Geometry: final body of the model. Coordinates: model frame, mm. A direction names the side the tool comes from. Give positions to 0.01 mm unless a question says otherwise; leave off trailing zeros. Order: outer loops, then holes, each group sorted by start corner. A loop starts at its lowest first (then second) coordinate and runs counter-clockwise, first axis right, second up. Notation, with made-up numbers: (89, 84.25) - (105, 84.25) arc R20 ccw to (105, 115.25) - close; hole circle Ø4 at (-15, 74). An arc over 180 degrees is marked (long way). One line per item, written item: value.
Autodesk Inventor part; units mm, degrees
ref_plane "Work Plane1" through (-25.4, 0, -5.08) normal (0, 0, 1) x (1, 0, 0)
ref_plane "YZ Plane" through (0, 0, 0) normal (1, 0, 0) x (0, 1, 0)
ref_plane "XZ Plane" through (0, 0, 0) normal (0, 1, 0) x (-1, 0, 0)
sketch "Sketch1" plane through (0, 0, 0) normal (0, 1, 0) x (-1, 0, 0)
  point P0 (0, 0)
sketch "Sketch2" plane through (0, 0, 0) normal (0, 1, 0) x (-1, 0, 0)
  line L0 (0, 0) -> (25.4, 0)
  line L1 (25.4, 0) -> (25.4, -50.8)
  line L2 (25.4, -50.8) -> (0, -50.8)
  line L3 (0, -50.8) -> (0, 0)
  dimension "d0" = 25.4
  dimension "d1" = 50.8
extrude "Extrusion1" add sketch "Sketch2" along normal blind 25.4
sketch "Sketch3" plane through (-25.4, 0, 0) normal (0, 0, 1) x (1, 0, 0)
  line L0 (0, 25.4) -> (25.4, 25.4)
  line L1 (0, 0) -> (0, 25.4)
  line L2 (25.4, 0) -> (25.4, 25.4)
  line L3 (3.81, 21.59) -> (21.59, 21.59)
  line L4 (21.59, 21.59) -> (21.59, 15.24)
  line L5 (21.59, 15.24) -> (3.81, 15.24)
  line L6 (3.81, 15.24) -> (3.81, 21.59)
  line L7 (25.4, 0) -> (0, 0)
  line L8 (3.81, 3.81) -> (21.59, 3.81)
  line L9 (21.59, 3.81) -> (21.59, 10.16)
  line L10 (21.59, 10.16) -> (3.81, 10.16)
  line L11 (3.81, 10.16) -> (3.81, 3.81)
  dimension "d4" = 3.81
  dimension "d5" = 3.81
  dimension "d6" = 3.81
  dimension "d7" = 6.35
  dimension "d8" = 3.81
  dimension "d9" = 6.35
extrude "Extrusion2" cut sketch "Sketch3" against normal blind 5.08 contours L3 L4 L5 L6 | L11 L10 L9 L8
ref_plane "Work Plane1" through (-25.4, 0, -5.08) normal (0, 0, 1) x (1, 0, 0)
sketch "Sketch4" plane through (-25.4, 0, -5.08) normal (0, 0, 1) x (1, 0, 0)
  line L0 (2.54, 22.86) -> (22.86, 22.86)
  line L1 (22.86, 22.86) -> (22.86, 2.54)
  line L2 (22.86, 2.54) -> (2.54, 2.54)
  line L3 (2.54, 2.54) -> (2.54, 22.86)
  line L4 (0, 25.4) -> (25.4, 25.4)
  line L5 (0, 0) -> (0, 25.4)
  line L6 (25.4, 0) -> (25.4, 25.4)
  line L7 (25.4, 0) -> (0, 0)
  dimension "d13" = 2.54
  dimension "d14" = 2.54
  dimension "d15" = 2.54
  dimension "d16" = 2.54
extrude "Extrusion3" cut sketch "Sketch4" against normal blind 43.18 contours L0 L1 L2 L3
sketch "Sketch5" plane through (0, 0, -50.8) normal (0, 0, -1) x (-1, 0, 0)
  line L0 (2.54, 2.54) -> (22.86, 2.54)
  line L1 (9.525, 8.89) -> (15.875, 8.89)
  line L2 (15.875, 8.89) -> (15.875, 2.54)
  line L3 (15.875, 2.54) -> (9.525, 2.54)
  line L4 (9.525, 2.54) -> (9.525, 8.89)
  line L5 (0, 0) -> (0, 25.4)
  dimension "d19" = 6.35
  dimension "d20" = 6.35
  dimension "d21" = 9.525
extrude "Extrusion4" cut sketch "Sketch5" against normal blind 12.7
sketch "Sketch6" plane through (-22.86, 2.54, -5.08) normal (1, 0, 0) x (0, 0, -1)
  line L0 (15.6891, 18.5897) -> (25.8491, 18.5897)
  line L1 (25.8491, 18.5897) -> (25.8491, 8.4297)
  line L2 (25.8491, 8.4297) -> (15.6891, 8.4297)
  line L3 (15.6891, 8.4297) -> (15.6891, 18.5897)
  point P0 (-5.08, -2.54)
  dimension "d24" = 10.16
  dimension "d25" = 10.16
extrude "Extrusion5" add sketch "Sketch6" along normal blind 5.08
sketch "Sketch7" plane through (-25.4, 0, -48.26) normal (0, 0, 1) x (1, 0, 0)
  line L0 (22.86, 2.54) -> (15.875, 2.54)
  line L1 (22.86, 22.86) -> (22.86, 2.54)
  circle A0 centre (19.8628, 5.54) radius 3
  point P0 (25.4, 0)
  dimension "d28" = 3
  dimension "d29" = 2.9972
  dimension "d30" = 6
extrude "Extrusion6" add sketch "Sketch7" along normal blind 33.02 contours A0 L1 | L1 A0
properties part number "sensor pod"
1) Material intervals for line 1 along Z through (x, y) = (-20, 15); line 2 along Y through (x, z) = (-22.5, -22.5); line 3 along Y through (x, z) = (-10, -5.5), sorted ascending.
Answers below:
line 1: -50.8 to -48.26, -30.93 to -20.77, -5.08 to 0
line 2: 0 to 2.54, 10.97 to 21.13, 22.86 to 25.4
line 3: 0 to 2.54, 22.86 to 25.4
2) Section B-B, the plane z = -11. Return loops of the section in (x, y).
Answers below:
outline: (-25.4, 0) - (0, 0) - (0, 25.4) - (-25.4, 25.4) - close; hole (-22.86, 2.54) - (-2.54, 2.54) - (-2.54, 22.86) - (-22.86, 22.86) - close
3) Mould query, pull axis X, two halves, no side actions, for faces 4 (the face through (-13, 13, -50.8)), 5 (the face through (-20, 16, -30.929)), 6 (the face through (0, 13, -26)). Classes: released by +X, released by -X, zero draft, split by the parting line, or undercut.
Answers below:
face 4: zero draft
face 5: undercut
face 6: released by +X
4) Section A-A, the plane y = 14.25. Return loops of the section in (x, z), then the cut area to 3 significant figures.
Answers below:
outline: (-25.4, -50.8) - (0, -50.8) - (0, 0) - (-25.4, 0) - close; hole (-22.86, -48.26) - (-2.54, -48.26) - (-2.54, -5.08) - (-22.86, -5.08) - (-22.86, -20.77) - (-17.78, -20.77) - (-17.78, -30.93) - (-22.86, -30.93) - close
area: 465 mm^2
5) Section C-C, the plane x = -6.5. Return loops of the section in (y, z).
Answers below:
outline: (0, -50.8) - (25.4, -50.8) - (25.4, 0) - (21.59, 0) - (21.59, -5.08) - (22.86, -5.08) - (22.86, -48.26) - (8.38, -48.26) - (8.38, -15.24) - (2.7, -15.24) - (2.7, -48.26) - (2.54, -48.26) - (2.54, -5.08) - (3.81, -5.08) - (3.81, 0) - (0, 0) - close; (10.16, -5.08) - (15.24, -5.08) - (15.24, 0) - (10.16, 0) - close
6) Set-up query: faces 1 (the face through (-17.78, 16, -26)), 2 (the face through (-9.525, 6, -50)), 3 (the face through (-13, 15.24, -3)). Return all of +Z, -Z, +X, -X, +Y, -Y with unobstructed straight access to the full face (end or side cutting, diameter ignored); none if empty.
Answers below:
face 1: none
face 2: -Z
face 3: +Z
